The model under review builds one solid part; all positions refer to its coordinate system, in mm. A direction names the side the tool comes from. Coordinates: 2 decimals unless noted, no trailing zeros. Order: outer loops, then holes, each group sorted by start corner. A loop starts at its lowest first (then second) coordinate and runs counter-clockwise, first axis right, second up. Notation, with made-up numbers: (48.25, 38) -> (94.25, 38) arc R33 cw to (94.25, 73) -> close; hole circle Ø3 at (75.25, 81.5). An arc over 180 degrees is marked (long way). Use one line per item in the form item = value. Start each with the question number.
(1) Take a section at D-D (x = -42). State the section outline as (y, z) points.
(2) Take a section at B-B (x = -151.5). State the section outline as (y, z) points.
(3) Insertion check: pin 1 Ø12.5 at (x, z) = (160.27, -12.7) entering from +Y; pin 2 Ø6 at (x, y) = (85, 284.5) entering from -Z. Each pin has a flat end and moves straight along its axis. Give the tip position at first contact, or say it passes through.
(4) Take a section at A-A (z = -21.75). State the section outline as (x, y) points.
(5) Take a section at C-C (y = 346). State the section outline as (x, z) points.
(6) Wall thickness on line 1 along X through (y, z) = (180.15, -12.7); line 2 along Z through (x, y) = (-141.5, 196); line 3 along Y through (x, z) = (-112, -1): over which ranges is each line inside the solid? List them lowest first.
(7) Mouldability with a two-part tool opening along Z and no side actions: class faces 1 (the cylindrical face through (155.51, 180.09, -12.91)), 2 (the flat face through (-133, 179.319, -12)), 3 (the flat face through (3, 250, 0)) as +Z half, -Z half, draft (parallel to the pull), parting line (faces both ways), or undercut.
(8) For faces 4 (the flat face through (3, 250, 1.519)), 5 (the flat face through (142, 180.838, -13)), list the 3-axis set-ups (+Z, -Z, +X, -X, +Y, -Y) from which the entire face can be reached by the end or side of a thin tool; tool diameter is ignored.
```python
from build123d import *

# Parameters (mm, degrees)
OUTER_CASING_DEPTH  = 1.51892
SKETCH1_R           = 15
INNER_CUTOUT_DEPTH  = 20
SKETCH4_W           = 76.2
SKETCH4_H           = 1.51892
BOSS_EXTRUDE1_DEPTH = 25.4
SKETCH5_R           = 4.7625
CUT_EXTRUDE1_DEPTH  = 2.51892


with BuildPart() as part:
    # Plate shape → Outer casing (new body)
    with BuildSketch(Plane.XY):
        with BuildLine():
            Line((0, 179.31892), (-179.31892, 179.31892))
            ThreePointArc((-179.31892, 179.31892), (0, 358.63784), (179.31892, 179.31892))
            Line((179.31892, 179.31892), (0, 179.31892))
        make_face()
    extrude(amount=OUTER_CASING_DEPTH)

    # Sketch1 → Inner Cutout (cut)
    with BuildSketch(Plane.XY.offset(1.51892)):
        with Locations((0, 179.31892)):
            Circle(SKETCH1_R)
    extrude(amount=-INNER_CUTOUT_DEPTH, mode=Mode.SUBTRACT)

    # Sketch4 → Boss-Extrude1 (add)
    with BuildSketch(Plane(origin=(0, 0, 0), x_dir=(-1, 0, 0), z_dir=(0, 0, -1))):
        with Locations((-141.21892, 180.07838)):
            Rectangle(SKETCH4_W, SKETCH4_H)
        with Locations((141.21892, 180.07838)):
            Rectangle(SKETCH4_W, SKETCH4_H)
    extrude(amount=BOSS_EXTRUDE1_DEPTH)

    # Sketch5 → Cut-Extrude1 (cut, through all)
    with BuildSketch(Plane(origin=(0, 180.83784, 0), x_dir=(1, 0, 0), z_dir=(0, 1, 0))):
        with Locations((160.26892, 12.7)):
            Circle(SKETCH5_R)
        with Locations((122.16892, 12.7)):
            Circle(SKETCH5_R)
        with Locations((-160.26892, 12.7)):
            Circle(SKETCH5_R)
        with Locations((-122.16892, 12.7)):
            Circle(SKETCH5_R)
    extrude(amount=-CUT_EXTRUDE1_DEPTH, mode=Mode.SUBTRACT)


solid = part.part
```
Findings:
q1.outline = (179.32, 0) -> (353.65, 0) -> (353.65, 1.52) -> (179.32, 1.52) -> close
q2.outline = (179.32, -25.4) -> (180.84, -25.4) -> (180.84, 0) -> (275.25, 0) -> (275.25, 1.52) -> (179.32, 1.52) -> close
q3.pin_1 = 180.84
q3.pin_2 = 0
q4.outline = (-179.32, 179.32) -> (-103.12, 179.32) -> (-103.12, 180.84) -> (-179.32, 180.84) -> close; (103.12, 179.32) -> (179.32, 179.32) -> (179.32, 180.84) -> (103.12, 180.84) -> close
q5.outline = (-66.13, 0) -> (66.13, 0) -> (66.13, 1.52) -> (-66.13, 1.52) -> close
q6.line_1 = -179.32 to -165.03, -155.51 to -126.93, -117.41 to -103.12, 103.12 to 117.41, 126.93 to 155.51, 165.03 to 179.32
q6.line_2 = 0 to 1.52
q6.line_3 = 179.32 to 180.84
q7.face_1 = undercut
q7.face_2 = draft
q7.face_3 = -Z half
q8.face_4 = +Z, +X, -X, +Y, -Y
q8.face_5 = -Z, +X, -X, +Y
